```python
from build123d import *

# Parameters (mm, degrees)
SKETCH_1_W          = 20
SKETCH_1_H          = 40
EXTRUDE_1_DEPTH     = 4
SKETCH_5_R          = 1.575
CUT_EXTRUDE_2_DEPTH = 45.899888641
EXTRUDE_2_DEPTH     = 4
SKETCH_11_R         = 2.6
CUT_EXTRUDE_3_DEPTH = 58.913728942
FILLET_1_R          = 4


with BuildPart() as part:
    # 草图1 → 凸台-拉伸1 (new body)
    with BuildSketch(Plane.XY):
        with Locations((10, -20)):
            Rectangle(SKETCH_1_W, SKETCH_1_H)
    extrude(amount=EXTRUDE_1_DEPTH)

    # 草图5 → 切除-拉伸2 (cut, through all)
    with BuildSketch(Plane.XY.offset(4)):
        with Locations((5, -5)):
            Circle(SKETCH_5_R)
        with Locations(Location((15, -5, 0), (0, 0, 180))):
            Circle(SKETCH_5_R)
        with Locations((15, -15)):
            Circle(SKETCH_5_R)
        with Locations(Location((5, -15, 0), (0, 0, 180))):
            Circle(SKETCH_5_R)
    extrude(amount=-CUT_EXTRUDE_2_DEPTH, mode=Mode.SUBTRACT)

    # 草图10 → 凸台-拉伸2 (add)
    with BuildSketch(Plane(origin=(0, 0, 0), x_dir=(-1, 0, 0), z_dir=(0, 0, -1))):
        Polygon((-23, -40), (-20, 0), (-20, -40), align=None)
        Polygon((0, -40), (3, -40), (0, 0), align=None)
        with BuildLine():
            Line((0, -40), (-20, -40))
            Line((-20, -40), (-23, -40))
            ThreePointArc((-23, -40), (-10, -53), (3, -40))
            Line((3, -40), (0, -40))
        make_face()
    extrude(amount=-EXTRUDE_2_DEPTH)

    # 草图11 → 切除-拉伸3 (cut, through all)
    with BuildSketch(Plane(origin=(0, 0, 0), x_dir=(-1, 0, 0), z_dir=(0, 0, -1))):
        with Locations((-10, -40)):
            Circle(SKETCH_11_R)
    extrude(amount=-CUT_EXTRUDE_3_DEPTH, mode=Mode.SUBTRACT)

    # 圆角1
    fillet_1_edges = [part.edges().sort_by_distance(p)[0] for p in [
        (0, 0, 2),
        (20, 0, 2),
    ]]
    fillet(fillet_1_edges, radius=FILLET_1_R)


solid = part.part
```
Model file for the job. Use its own axes, mm. Give positions to 0.01 mm unless a question says otherwise; leave off trailing zeros. Order: outer loops, then holes, each group sorted by start corner. A loop starts at its lowest first (then second) coordinate and runs counter-clockwise, first axis right, second up.
1) Pin check, flat tips, straight feed: pin 1 (5 mm diameter, centred on x = 5, y = -5, fed in from +Z); pin 2 (1.5 mm diameter, centred on x = 20.5, z = 1.5, fed in from -Y). Stop position of each tip, or through.
2) Saw through at C-C, the plane x = 10. Write the cut outline in (y, z).
3) Saw through at D-D, the plane y = -15. Write the cut outline in (x, z) (3 decimals).
4) Mould opens along X. For faces 1 (the cylindrical face through (3.839, -3.936, 2.028)), 2 (the cylindrical face through (10, -53, 2)), 3 (the cylindrical face through (1.02, -1.04, 2.03)) say: +X half, -X half, draft (parallel to the pull), parting line (faces both ways), or undercut.
5) Saw through at B-B, the plane z = 1.7. Write the cut outline in (x, y) (3 decimals).
6) Saw through at A-A, the plane x = 15. Write the cut outline in (y, z) (3 decimals).
7) Wall check: probe 1 along X at (y, z) = (-6, 3.3); probe 2 along Y at (x, z) = (15, 3.1) (3 decimals); probe 3 along Y at (x, z) = (14, 3.45). Give the ranges that are in metal, low to high.
Computed:
1. pin 1: stops at z = 4
1. pin 2: stops at y = -48.6
2. outline: (-53, 0) - (-42.6, 0) - (-42.6, 4) - (-53, 4) - close; (-37.4, 0) - (0, 0) - (0, 4) - (-37.4, 4) - close
3. outline: (-1.125, 0) - (3.425, 0) - (3.425, 4) - (-1.125, 4) - close; (6.575, 0) - (13.425, 0) - (13.425, 4) - (6.575, 4) - close; (16.575, 0) - (21.125, 0) - (21.125, 4) - (16.575, 4) - close
4. face 1: undercut
4. face 2: parting line
4. face 3: -X half
5. outline: (-3, -40) arc R13 ccw to (23, -40) - (20.278, -3.701) arc R4 ccw to (16.289, 0) - (3.711, 0) arc R4 ccw to (-0.278, -3.701) - close; hole circle Ø3.15 at (5, -15); hole circle Ø3.15 at (5, -5); hole circle Ø5.2 at (10, -40); hole circle Ø3.15 at (15, -15); hole circle Ø3.15 at (15, -5)
6. outline: (-52, 0) - (-16.575, 0) - (-16.575, 4) - (-52, 4) - close; (-13.425, 0) - (-6.575, 0) - (-6.575, 4) - (-13.425, 4) - close; (-3.425, 0) - (0, 0) - (0, 4) - (-3.425, 4) - close
7. probe 1: x = -0.45 to 3.78, 6.22 to 13.78, 16.22 to 20.45
7. probe 2: y = -52 to -16.575, -13.425 to -6.575, -3.425 to 0
7. probe 3: y = -52.37 to -16.22, -13.78 to -6.22, -3.78 to 0
